Verification items for the finished model (mm, model axes). A direction names the side the tool comes from. Coordinates: 2 decimals unless noted, no trailing zeros. Order: outer loops, then holes, each group sorted by start corner. A loop starts at its lowest first (then second) coordinate and runs counter-clockwise, first axis right, second up. Notation, with made-up numbers: (-3, -39.75) - (39, -39.75) arc R19 cw to (39, -2.75) - close; hole circle Ø5 at (28.5, 86.25). An arc over 180 degrees is marked (long way). One line per question, with ' | ' between items. Start each with the question number.
from build123d import *

# Parameters (mm, degrees)
F0_R     = 3.5
F0_R_2   = 2
F1_DEPTH = 4
F2_DEPTH = 70
F3_DEPTH = 1.5
F4_R     = 0.2


with BuildPart() as f1:
    # F0 (on Top) → F1 (new body)
    with BuildSketch(Plane.XY):
        Circle(F0_R)
        Circle(F0_R_2, mode=Mode.SUBTRACT)
        Circle(F0_R_2)
        Polygon((0, 1.732051), (1.5, 0.866025), (1.5, -0.866025), (0, -1.732051), (-1.5, -0.866025), (-1.5, 0.866025), align=None, mode=Mode.SUBTRACT)
    extrude(amount=F1_DEPTH)

    # F0 (on Top) → F2 (join)
    with BuildSketch(Plane.XY):
        Circle(F0_R_2)
        Polygon((0, 1.732051), (1.5, 0.866025), (1.5, -0.866025), (0, -1.732051), (-1.5, -0.866025), (-1.5, 0.866025), align=None, mode=Mode.SUBTRACT)
        Polygon((1.5, -0.866025), (1.5, 0.866025), (0, 1.732051), (-1.5, 0.866025), (-1.5, -0.866025), (0, -1.732051), align=None)
    extrude(amount=-F2_DEPTH)

    # F0 (on Top) → F3 (join)
    with BuildSketch(Plane.XY):
        Polygon((1.5, -0.866025), (1.5, 0.866025), (0, 1.732051), (-1.5, 0.866025), (-1.5, -0.866025), (0, -1.732051), align=None)
    extrude(amount=F3_DEPTH)

    # F4
    f4_edges = [f1.edges().sort_by_distance(p)[0] for p in [
        (-3.5, 0, 4),
        (-0.75, -1.299038, 4),
        (-1.5, 0, 4),
        (-0.75, 1.299038, 4),
        (0.75, 1.299038, 4),
        (1.5, 0, 4),
        (0.75, -1.299038, 4),
    ]]
    fillet(f4_edges, radius=F4_R)


solid = f1.part
Item 1: Mould release check, pull along X, two halves, no side actions. Record for faces 4 (the flat face through (0.74, 1.305, 2.634)), 5 (the flat face through (0, 0, -70)), 6 (the cylindrical face through (0, -2, -35)), 7 (the flat face through (-0.74, -1.305, 2.634)): +X half, -X half, draft (parallel to the pull), parting line (faces both ways), or undercut.
Item 2: Set-up check for faces 1 (the flat face through (0.76, -1.293, 2.634)), 2 (the flat face through (2, -2, 0)), 3 (the cylindrical face through (3.233, -1.341, 1.873)): record each of +Z, -Z, +X, -X, +Y, -Y from which the full face is reachable in a straight line by a thin tool's end or side.
Item 3: Section check B-B (z = -33.5). Record the cut outline in (x, y), then the cut area to 3 significant figures.
Item 4: Thickness scan on probe 1 along Y at (x, z) = (0.25, -53); probe 2 along X at (y, z) = (-1.75, -65.5); probe 3 along Z at (x, y) = (-2, -1.75). Record the ranges inside material, lowest first. Write a range as from..to.
Item 5: Section check A-A (y = 0). Record the cut outline in (x, z), then the cut area to 3 significant figures.
Item 6: Gauge pin test, flat ends, axial feed: pin 1 (4 mm diameter, centred on x = 1, z = -30.5, fed in from +Y); pin 2 (1.5 mm diameter, centred on y = -2.5, z = -40.5, fed in from -X); pin 3 (0.5 mm diameter, centred on y = -0.5, z = 2.5, fed in from -X). Record the tip position at first contact, or that the pin passes through.
Completed:
1) face 4: undercut | face 5: draft | face 6: parting line | face 7: undercut
2) face 1: +Z | face 2: -Z | face 3: +Z, -Z
3) outline: circle Ø4 at (0, 0) | area: 12.6 mm^2
4) probe 1: y = -1.98..1.98 | probe 2: x = -0.97..0.97 | probe 3: z = 0..4
5) outline: (-3.5, 0) - (-2, 0) - (-2, -70) - (2, -70) - (2, 0) - (3.5, 0) - (3.5, 3.8) arc R0.2 ccw to (3.3, 4) - (1.7, 4) arc R0.2 ccw to (1.5, 3.8) - (1.5, 1.5) - (-1.5, 1.5) - (-1.5, 3.8) arc R0.2 ccw to (-1.7, 4) - (-3.3, 4) arc R0.2 ccw to (-3.5, 3.8) - close | area: 300 mm^2
6) pin 1: stops at y = 2 | pin 2: stops at x = -0.97 | pin 3: stops at x = -3.49
